Build history of the part. All positions in model axes, mm. A direction names the side the tool comes from. Give positions to 0.01 mm unless a question says otherwise; leave off trailing zeros. Order: outer loops, then holes, each group sorted by start corner. A loop starts at its lowest first (then second) coordinate and runs counter-clockwise, first axis right, second up. Notation, with made-up numbers: M 30,-22 L 40,-22 A22 cw 40,17 Z; hole C -37,68.5 d5. An arc over 180 degrees is marked long. One line per item, written item: value. Start each with the question number.
from build123d import *

# Parameters (mm, degrees)
WYCI_GNI_CIE_CIENKA_CIANKA1_DEPTH = 102
OTW_R1_D                          = 6
OTW_R1_DEPTH                      = 1
OTW_R2_D                          = 6
OTW_R2_DEPTH                      = 1
ZAOKR_GLENIE1_R                   = 5
OTW_R3_D                          = 6
OTW_R3_DEPTH                      = 1
OTW_R4_D                          = 6
OTW_R4_DEPTH                      = 1


with BuildPart() as part:
    # Szkic1 → Wyciągnięcie-cienka ścianka1 (new body)
    with BuildSketch(Plane.XY):
        with BuildLine():
            Line((134.043918698, -128), (129.158561205, 40.663670642))
            ThreePointArc((129.158561205, 40.663670642), (101.302286813, 103.988853979), (37.19712984, 130))
            Line((37.19712984, 130), (-9.80287016, 130))
            ThreePointArc((-9.80287016, 130), (-109.26340878, 82.570473856), (-135.015100263, -24.568730353))
            Line((-135.015100263, -24.568730353), (-111.522833189, -135.282306482))
            Line((-111.522833189, -135.282306482), (-112.501053736, -135.489874688))
            Line((-112.501053736, -135.489874688), (-135.993320811, -24.776298559))
            ThreePointArc((-135.993320811, -24.776298559), (-110.040444238, 83.199930683), (-9.80287016, 131))
            Line((-9.80287016, 131), (37.19712984, 131))
            ThreePointArc((37.19712984, 131), (101.999081998, 104.706124131), (130.158141981, 40.692623583))
            Line((130.158141981, 40.692623583), (135.043499474, -127.971047058))
            Line((135.043499474, -127.971047058), (134.043918698, -128))
        make_face()
    extrude(amount=WYCI_GNI_CIE_CIENKA_CIANKA1_DEPTH)

    # Otwór1
    with Locations(Plane(origin=(131.226711189, 3.800992794, 0), x_dir=(0, 0, -1), z_dir=(0.999580776, 0.028952942, 0))):
        with Locations((-78, -121.827305061)):
            Hole(OTW_R1_D / 2, depth=OTW_R1_DEPTH)

    # Otwór2
    with Locations(Plane(origin=(131.226711189, 3.800992794, 0), x_dir=(0, 0, -1), z_dir=(0.999580776, 0.028952942, 0))):
        with Locations((-24, -121.827305061)):
            Hole(OTW_R2_D / 2, depth=OTW_R2_DEPTH)

    # Zaokrąglenie1
    zaokr_glenie1_edges = [part.edges().sort_by_distance(p)[0] for p in [
        (134.543709086, -127.985523529, 0),
        (-112.011943462, -135.386090585, 0),
        (134.543709086, -127.985523529, 102),
        (-112.011943462, -135.386090585, 102),
    ]]
    fillet(zaokr_glenie1_edges, radius=ZAOKR_GLENIE1_R)

    # Otwór3
    with Locations(Plane(origin=(-135.164873494, -28.680577561, 0), x_dir=(0, 0, 1), z_dir=(-0.978220548, -0.207568206, 0))):
        with Locations((24, -99.187337539)):
            Hole(OTW_R3_D / 2, depth=OTW_R3_DEPTH)

    # Otwór4
    with Locations(Plane(origin=(-135.164873494, -28.680577561, 0), x_dir=(0, 0, 1), z_dir=(-0.978220548, -0.207568206, 0))):
        with Locations((78, -99.187337539)):
            Hole(OTW_R4_D / 2, depth=OTW_R4_DEPTH)


solid = part.part
1) Slice it at B-B (y = 59). List the corners of the cut face in (x, z), plus the area to 3 significant figures.
2) Drop flat-ended pins along their axis: P1, Ø12, axis at x = 86.5, z = 64.5, coming from the +Y side; P2, Ø4, axis at y = -1.5, z = 37.5, coming from the -X side; P3, Ø2, axis at y = -77, z = 68.5, coming from the -X side. Give the stop position or say it passes through.
3) Slice it at C-C (y = -57.5). List the corners of the cut face in (x, z), plus the area to 3 significant figures.
4) Slice it at D-D (x = 48). List the corners of the cut face in (y, z).
5) Tool access for faces 1 (the flat face through (-123.433, -79.151, 50.286)), 2 (the flat face through (13, 131, 50)), 3 (the flat face through (14, 130, 50)), 4 (the cylindrical face through (-114.5, -123.62, 26.21)): list every direction of +Z, -Z, +X, -X, +Y, -Y with a clear straight run to the whole face (end or side of a thin tool).
6) Drill centre lines: line 1 (X direction, y = 67.5, z = 11.5); line 2 (X direction, y = 89, z = 59.5); line 3 (Y direction, x = 63, z = 51.5). Where is each one in solid material? Low to high.
7) Slice it at A-A (z = 39). List the corners of the cut face in (x, y).
8) Pull direction Y, two halves, no side cores. Call faces 5 (the cylindrical face through (101.275, 105.402, 50.286)), 6 (the cylindrical face through (-108.252, 83.803, 50.286)), 7 (the flat face through (-124.083, -80.908, 50.286)): pulls with the +Y half, pulls with the -Y half, needs draft (parallel to the pull), parting line crosses it, or undercut.
Results list:
1. outline: M -125.53,0 L -124.41,0 L -124.41,102 L -125.53,102 Z; M 126.77,0 L 127.8,0 L 127.8,102 L 126.77,102 Z
1. area: 219 mm²
2. P1: stops at y = 120.3
2. P2: stops at x = -138.79
2. P3: stops at x = -125.12
3. outline: M -129.05,0 L -128.03,0 L -128.03,102 L -129.05,102 Z; M 132,0 L 133,0 L 133,102 L 132,102 Z
3. area: 206 mm²
4. outline: M 129.36,0 L 130.37,0 L 130.37,102 L 129.36,102 Z
5. face 1: +Z, -Z
5. face 2: +Z, -Z, +X, -X, +Y
5. face 3: +Z, -Z, -Y
5. face 4: none
6. line 1: x = -120.94 to -119.77, 124.34 to 125.39
6. line 2: x = -105.05 to -103.69, 113.77 to 114.97
6. line 3: y = 126.31 to 127.35
7. outline: M -135.99,-24.78 L -112.5,-135.49 L -111.52,-135.28 L -135.02,-24.57 A128 cw -9.8,130 L 37.2,130 A92 cw 129.16,40.66 L 134.04,-128 L 135.04,-127.97 L 130.16,40.69 A93 ccw 37.2,131 L -9.8,131 A129 ccw Z
8. face 5: pulls with the +Y half
8. face 6: undercut
8. face 7: pulls with the -Y half
